Geometry: see drawing. Coordinates: mm, zero at the bounding-box minimum. A direction names the side the tool comes from. Give positions to 0.01 mm unless a question says otherwise; leave off trailing zeros. Write each loop counter-clockwise with the first axis right and the second up, starting at its lowest first coordinate (ties: lowest second). Pieces come first, ordered by that corner, then holes. Notation, with made-up numbers: (62, 64.25) - (102, 64.25) arc R19 ccw to (102, 79.25) - close; hole circle Ø3 at (13.25, 80.25). An arc over 180 degrees is marked (long way). Return JSON: item names as keys, results as strings.
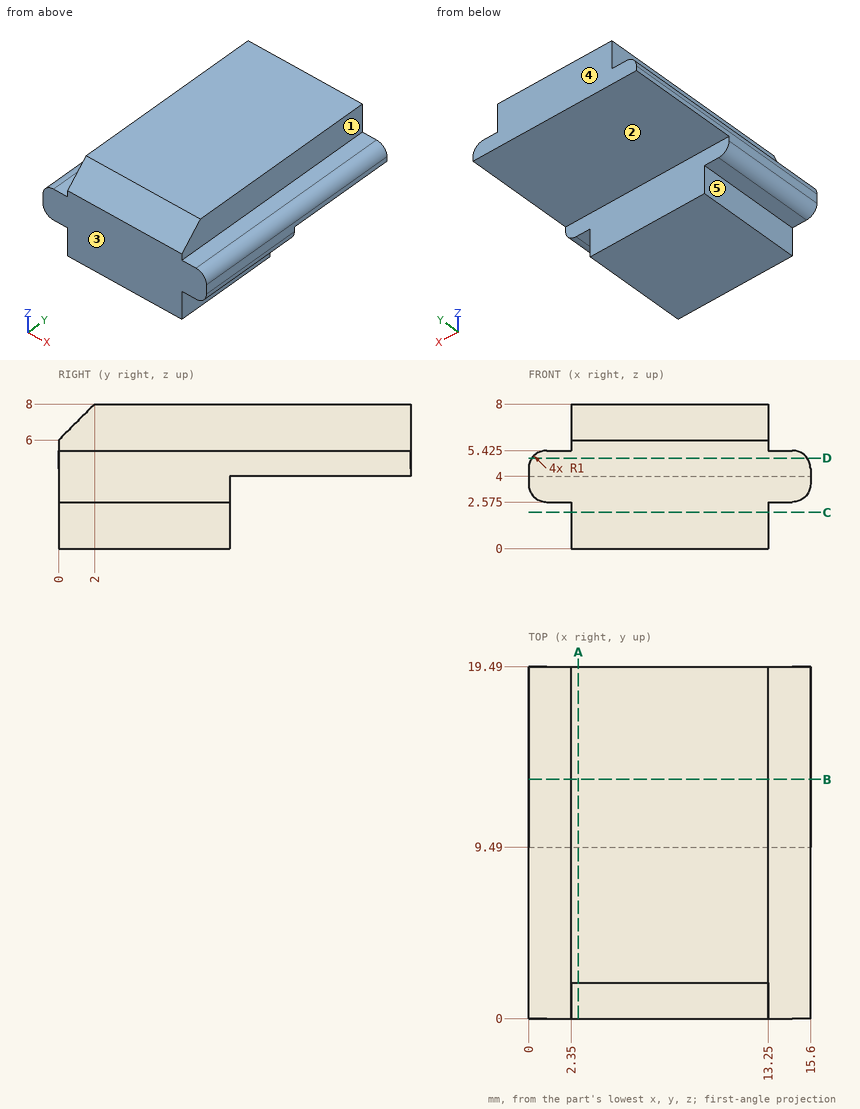
Q1. Set-up query: the marked faces 1, 2, 3, 4 and 5. Return all of +Z, -Z, +X, -X, +Y, -Y with unobstructed straight access to the full face (end or side cutting, diameter ignored); none if empty.
Answer key:
{"face 1": "+Z, +X, +Y, -Y", "face 2": "-Z, +X, -X, +Y", "face 3": "+Z, -Z, +X, -X, -Y", "face 4": "+Z, -Z, +X, -X, +Y", "face 5": "-Z, -X, +Y, -Y"}
Q2. Pin query (flat end, axial travel): P1, Ø1.1, axis at x = 13.5, y = 7, coming from the -Z side; P2, Ø2, axis at y = 9.5, z = 7, coming from the -X side; P3, Ø2, axis at x = 4.5, z = 2.5, coming from the +Y side; P4, Ø2, axis at y = 4.5, z = 1, coming from the +X side. Return the tip coordinate at first contact, or that it passes through.
Answer key:
{"P1": "stops at z = 0", "P2": "stops at x = 2.35", "P3": "stops at y = 9.49", "P4": "stops at x = 13.25"}
Q3. Section query D-D, the plane z = 5. Return the cut outline in (x, y), plus the area to 3 significant figures.
Answer key:
{"outline": "(0.18, 0) - (15.42, 0) - (15.42, 19.49) - (0.18, 19.49) - close", "area": "297 mm^2"}
Q4. Section query C-C, the plane z = 2. Return the cut outline in (x, y), plus the area to 3 significant figures.
Answer key:
{"outline": "(2.35, 0) - (13.25, 0) - (13.25, 9.49) - (2.35, 9.49) - close", "area": "103 mm^2"}
Q5. Section query B-B, the plane y = 13.25. Return the cut outline in (x, z) (3 decimals).
Answer key:
{"outline": "(0, 4) - (15.6, 4) - (15.6, 4.425) arc R1 ccw to (14.6, 5.425) - (13.25, 5.425) - (13.25, 8) - (2.35, 8) - (2.35, 5.425) - (1, 5.425) arc R1 ccw to (0, 4.425) - close"}
Q6. Material intervals for probe 1 along X at (y, z) = (4.5, 5.5); probe 2 along Y at (x, z) = (10.25, 3.75); probe 3 along Z at (x, y) = (12, 11), sorted ascending. Write a range as [from, to].
Answer key:
{"probe 1": "x = [2.35, 13.25]", "probe 2": "y = [0, 9.49]", "probe 3": "z = [4, 8]"}
Q7. Section query A-A, the plane x = 2.75. Return the cut outline in (y, z).
Answer key:
{"outline": "(0, 0) - (9.49, 0) - (9.49, 4) - (19.49, 4) - (19.49, 8) - (2, 8) - (0, 6) - close"}
